Geometry check sheet. Reference: the model listing, model coordinates, mm. Coordinates: 2 decimals unless noted, no trailing zeros. Order: outer loops, then holes, each group sorted by start corner. A loop starts at its lowest first (then second) coordinate and runs counter-clockwise, first axis right, second up. Notation, with made-up numbers: M 67.5,87 L 101.5,87 A31 cw 101.5,124 Z; hole C -11.5,48.5 d5. An arc over 180 degrees is marked long. One line per item, written item: value. Start each with the question number.
1) Sectioned sample at A-A, the plane z = 92.75. Enter the section's corners in (x, y), then the cut area to 3 significant figures.
2) Thickness scan on L1, parallel to Y at x = 712, z = 94.25; L2, parallel to X at y = -229, z = 90; L3, parallel to X at y = -206, z = 94.75. Record the ranges inside material, lowest first. Write a range as from..to.
3) Sectioned sample at B-B, the plane y = -219. Enter the section's corners in (x, z) (3 decimals), then the cut area to 3 significant figures.
4) Go/stop test with a flat-tipped pin: P1, Ø1.5, axis at y = -220, z = 90.5, coming from the -X side. Record where the tip stops, or that it passes through.
5) Sectioned sample at C-C, the plane x = 688. Enter the section's corners in (y, z) (3 decimals).
```python
from build123d import *

# Parameters (mm, degrees)
BOSS_EXTRUDE1_DEPTH = 3.175


with BuildPart() as part:
    # Sketch1 → Boss-Extrude1 (new, symmetric)
    with BuildSketch(Plane.XY.offset(93)):
        with BuildLine():
            Line((786.672833799, -234.297326982), (778.40142943, -234.297326982))
            Line((778.40142943, -234.297326982), (751.84, -207.735897552))
            ThreePointArc((751.84, -207.735897552), (750.191929388, -206.634691975), (748.247897552, -206.248))
            Line((748.247897552, -206.248), (667.381261469, -206.248))
            Line((667.381261469, -206.248), (678.811261469, -194.818))
            Line((678.811261469, -194.818), (793.814823755, -194.818))
            Line((793.814823755, -194.818), (795.830241145, -206.248))
            Line((795.830241145, -206.248), (791.618686937, -206.248))
            Line((791.618686937, -206.248), (786.672833799, -234.297326982))
        make_face()
    extrude(amount=BOSS_EXTRUDE1_DEPTH, both=True)


solid = part.part
```
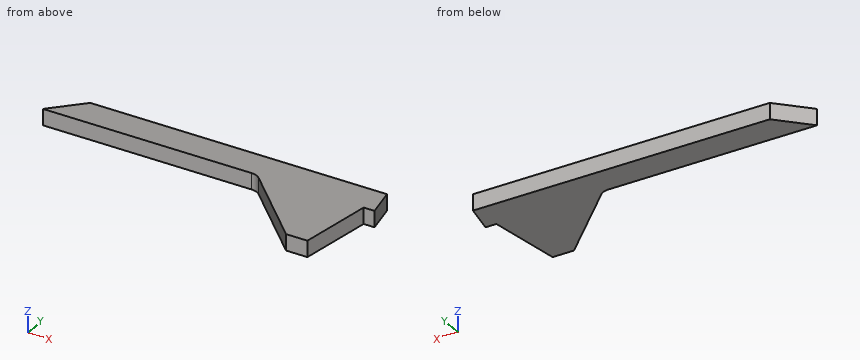
Final values:
1. outline: M 667.38,-206.25 L 748.25,-206.25 A5.08 cw 751.84,-207.74 L 778.4,-234.3 L 786.67,-234.3 L 791.62,-206.25 L 795.83,-206.25 L 793.81,-194.82 L 678.81,-194.82 Z
1. area: 2,090 mm^2
2. L1: y = -206.25..-194.82
2. L2: x = 773.1..787.61
2. L3: x = 667.63..795.79
3. outline: M 763.104,89.825 L 789.37,89.825 L 789.37,96.175 L 763.104,96.175 Z
3. area: 167 mm^2
4. P1: stops at x = 763.35
5. outline: M -206.248,89.825 L -194.818,89.825 L -194.818,96.175 L -206.248,96.175 Z
